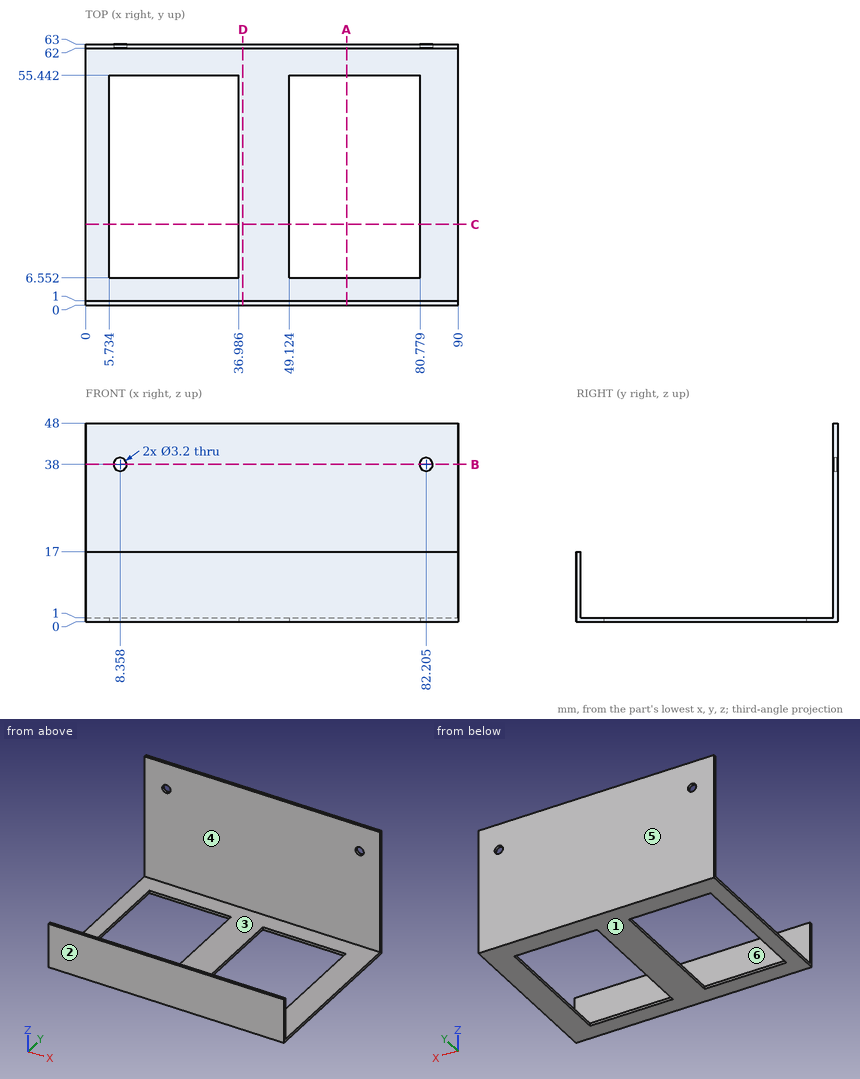
Source: three-view drawing plus pictorial views. Frame: mm from the lowest corner of the part. A direction names the side the tool comes from. Give positions to 0.01 mm unless a question says otherwise; leave off trailing zeros. Loops run counter-clockwise (first coordinate to the right, second up) from the corner with the lowest first, then second, coordinate; pieces in that order, holes last. Notation, with made-up numbers: M 22.5,23.5 L 27.5,23.5 A12 ccw 27.5,34.5 Z; hole C 43.5,55 d10. An arc over 180 degrees is marked long. Use CSV: the item, a comma, the result in double quotes.
(1) Section D-D, the plane x = 38. Return loops of the section in (y, z), plus the area to 3 significant figures.
Outcome:
outline,"M 0,0 L 63,0 L 63,48 L 62,48 L 62,1 L 1,1 L 1,17 L 0,17 Z"
area,"126 mm²"
(2) Pin query (flat end, axial travel): P1, Ø5, axis at x = 49.5, y = 12, coming from the +Z side; P2, Ø1, axis at x = 38, z = 15, coming from the -Y side; P3, Ø3, axis at x = 57, z = 36.5, coming from the -Y side; P4, Ø8, axis at x = 17, y = 47.5, coming from the +Z side. Return the tip coordinate at first contact, or that it passes through.
Outcome:
P1,"stops at z = 1"
P2,"stops at y = 0"
P3,"stops at y = 62"
P4,"passes through"
(3) Set-up query: the marked faces 5 and 6. Return all of +Z, -Z, +X, -X, +Y, -Y with unobstructed straight access to the full face (end or side cutting, diameter ignored); none if empty.
Outcome:
face 5,"+Z, -Z, +X, -X, +Y"
face 6,"+Z, +X, -X"
(4) Section A-A, the plane x = 63. Return loops of the section in (y, z).
Outcome:
outline,"M 0,0 L 6.55,0 L 6.55,1 L 1,1 L 1,17 L 0,17 Z; M 55.44,0 L 63,0 L 63,48 L 62,48 L 62,1 L 55.44,1 Z"
(5) Section B-B, the plane z = 38. Return loops of the section in (x, y) (1 decimal).
Outcome:
outline,"M 0,62 L 6.8,62 L 6.8,63 L 0,63 Z; M 10,62 L 80.6,62 L 80.6,63 L 10,63 Z; M 83.8,62 L 90,62 L 90,63 L 83.8,63 Z"
(6) Pull-direction query (Y, two-part tool) for the marked faces 1, 2, 3 and 4; classes: pulls with the +Y half, pulls with the -Y half, needs draft (parallel to the pull), parting line crosses it, or undercut.
Outcome:
face 1,"needs draft"
face 2,"pulls with the -Y half"
face 3,"undercut"
face 4,"undercut"
(7) Section C-C, the plane y = 19.5. Return loops of the section in (x, z) (1 decimal).
Outcome:
outline,"M 0,0 L 5.7,0 L 5.7,1 L 0,1 Z; M 37,0 L 49.1,0 L 49.1,1 L 37,1 Z; M 80.8,0 L 90,0 L 90,1 L 80.8,1 Z"
(8) Material intervals for L1, parallel to X at y = 62.5, z = 38 (1 decimal); L2, parallel to Y at x = 57, z = 15.5; L3, parallel to Y at x = 74.5, z = 29.5, sorted ascending. Write a range as [from, to].
Outcome:
L1,"x = [0, 6.8], [10, 80.6], [83.8, 90]"
L2,"y = [0, 1], [62, 63]"
L3,"y = [62, 63]"
